```python
from build123d import *

# Parameters (mm, degrees)
SKETCH_1_R          = 1.75
EXTRUDE_1_DEPTH     = 2
SKETCH_2_R          = 4.75
CUT_EXTRUDE_1_DEPTH = 2


with BuildPart() as part:
    # 草图1 → 凸台-拉伸1 (new body)
    with BuildSketch(Plane.XY):
        with BuildLine():
            Line((-50, 4.5), (-8.354386795, 7.90279832))
            ThreePointArc((-8.354386795, 7.90279832), (11.5, 0), (-8.354386795, -7.90279832))
            Line((-8.354386795, -7.90279832), (-50, -4.5))
            ThreePointArc((-50, -4.5), (-54.5, 0), (-50, 4.5))
        make_face()
        with Locations((-50, 0)):
            Circle(SKETCH_1_R, mode=Mode.SUBTRACT)
        with Locations((4.949747468, 4.949747468)):
            Circle(SKETCH_1_R, mode=Mode.SUBTRACT)
        with Locations((4.949747468, -4.949747468)):
            Circle(SKETCH_1_R, mode=Mode.SUBTRACT)
        with Locations((-4.949747468, -4.949747468)):
            Circle(SKETCH_1_R, mode=Mode.SUBTRACT)
        with Locations((-4.949747468, 4.949747468)):
            Circle(SKETCH_1_R, mode=Mode.SUBTRACT)
    extrude(amount=EXTRUDE_1_DEPTH)

    # 草图2 → 切除-拉伸1 (cut)
    with BuildSketch(Plane.XY.offset(2)):
        Circle(SKETCH_2_R)
    extrude(amount=-CUT_EXTRUDE_1_DEPTH, mode=Mode.SUBTRACT)


solid = part.part
```
Source: CAD feature listing. Evaluate the final solid. Frame: model axes, mm. Coordinates: 2 decimals unless noted, no trailing zeros. Loops run counter-clockwise (first coordinate to the right, second up) from the corner with the lowest first, then second, coordinate; pieces in that order, holes last. Notation, with made-up numbers: M -20.5,66 L 25.5,66 A15 ccw 25.5,87 Z; hole C 21,42 d6. An arc over 180 degrees is marked long. Use a Markdown table: item, result. Add a question column.
Q1. Section query D-D, the plane y = 9.25. Return loops of the section in (x, z), and give its area (3 significant figures).
Q2. Draft query along Y for faces 1 (the flat face through (-28.886, -6.225, 0.986)), 2 (the flat face through (-14, 0, 2)), 3 (the cylindrical face through (-6.338, 3.885, 0.986)). Return one class per face: pulls with the +Y half, pulls with the -Y half, needs draft (parallel to the pull), parting line crosses it, or undercut.
Q3. First-contact query: pin 1 (3 mm diameter, centred on x = -4.95, y = -4.95, fed in from +Z); pin 2 (1 mm diameter, centred on y = -2, z = 1.5, fed in from +X). Flat tips, straight axial feed; report the tip coordinate or a pass-through.
Q4. Section query C-C, the plane x = -21. Return loops of the section in (y, z), and give its area (3 significant figures).
Q5. Section query B-B, the plane y = 0. Return loops of the section in (x, z).
Q6. Section query A-A, the plane x = 0. Return loops of the section in (y, z).
Q7. Material intervals for L1, parallel to Y at x = -50, z = 1; L2, parallel to X at y = -0.75, z = 0.55; L3, parallel to Y at x = 0, z = 0.6, sorted ascending.
Result:
| question | item | result |
|---|---|---|
| 1 | outline | M -6.83,0 L 6.83,0 L 6.83,2 L -6.83,2 Z |
| 1 | area | 27.3 mm2 |
| 2 | face 1 | pulls with the -Y half |
| 2 | face 2 | needs draft |
| 2 | face 3 | undercut |
| 3 | pin 1 | passes through |
| 3 | pin 2 | stops at x = 11.4 |
| 4 | outline | M -6.87,0 L 6.87,0 L 6.87,2 L -6.87,2 Z |
| 4 | area | 27.5 mm2 |
| 5 | outline | M -54.5,0 L -51.75,0 L -51.75,2 L -54.5,2 Z; M -48.25,0 L -4.75,0 L -4.75,2 L -48.25,2 Z; M 4.75,0 L 11.5,0 L 11.5,2 L 4.75,2 Z |
| 6 | outline | M -11.5,0 L -4.75,0 L -4.75,2 L -11.5,2 Z; M 4.75,0 L 11.5,0 L 11.5,2 L 4.75,2 Z |
| 7 | L1 | y = -4.5 to -1.75, 1.75 to 4.5 |
| 7 | L2 | x = -54.44 to -51.58, -48.42 to -4.69, 4.69 to 11.48 |
| 7 | L3 | y = -11.5 to -4.75, 4.75 to 11.5 |
